Geometry check sheet. Reference: the model listing, model coordinates, mm. Round coordinates to 2 decimals unless told otherwise and drop trailing zeros. Write each loop counter-clockwise with the first axis right and the second up, starting at its lowest first coordinate (ties: lowest second). Pieces come first, ordered by that corner, then holes. Notation, with made-up numbers: M 43,54 L 68,54 A4 cw 68,58 Z; hole C 21,66 d7. An arc over 180 degrees is marked long. Put each result on its own line as item: value. Start each with the question number.
(1) Mould release check, pull along X, two halves, no side actions. Record for faces 1 (the flat face through (18, 1, 3.18)), 2 (the cylindrical face through (-0.54, -2.44, 1.61)): pulls with the +X half, pulls with the -X half, needs draft (parallel to the pull), parting line crosses it, or undercut.
(2) Section check A-A on z = 0.85. Count the separate pieces of the cut face and the enclosed holes in it, then the cut area to 3 significant figures.
(3) Material ranges on probe 1 along Y at (x, z) = (-70, 3.05); probe 2 along Y at (x, z) = (6.1, 1.55); probe 3 along Y at (x, z) = (2, 1), recorded low to high.
(4) Section check B-B on x = 36. Record the cut outline in (y, z).
(5) Gauge pin test, flat ends, axial feed: pin 1 (0.9 mm diameter, centred on x = -69, z = 2, fed in from -Y); pin 2 (1.6 mm diameter, centred on x = -77, z = 2, fed in from +Y); pin 3 (1.5 mm diameter, centred on y = -3.5, z = 1, fed in from +X). Record the tip position at first contact, or that the pin passes through.
from build123d import *

# Parameters (mm, degrees)
SKETCH1_R           = 1.5
BOSS_EXTRUDE1_DEPTH = 3.18
SKETCH2_R           = 2.5
SKETCH2_R_2         = 1.5
CUT_EXTRUDE1_DEPTH  = 20
SKETCH3_R           = 1.5
CUT_EXTRUDE2_DEPTH  = 20
SKETCH5_R           = 1.5
CUT_EXTRUDE4_DEPTH  = 4


with BuildPart() as part:
    # Sketch1 → Boss-Extrude1 (new body)
    with BuildSketch(Plane.XY):
        Polygon((-78.18, 75), (-12.5, 75), (-12.5, 78.18), (12.5, 78.18), (12.5, 75), (78.18, 75), (78.18, 12.5), (75, 12.5), (75, 1.5), (71, 1.5), (71, 4.5), (68, 4.5), (68, 1.5), (65.18, 1.5), (65.18, -1.5), (68, -1.5), (68, -4.5), (71, -4.5), (71, -1.5), (75, -1.5), (75, -12.5), (78.18, -12.5), (78.18, -75), (12.5, -75), (12.5, -78.18), (-12.5, -78.18), (-12.5, -75), (-78.18, -75), (-78.18, -12.5), (-75, -12.5), (-75, -1.5), (-71, -1.5), (-71, -4.5), (-68, -4.5), (-68, -1.5), (-65.18, -1.5), (-65.18, 1.5), (-68, 1.5), (-68, 4.5), (-71, 4.5), (-71, 1.5), (-75, 1.5), (-75, 12.5), (-78.18, 12.5), align=None)
        with Locations(Location((0, -76.59, 0), (0, 0, 180))):
            Circle(SKETCH1_R, mode=Mode.SUBTRACT)
        with Locations(Location((0, 76.59, 0), (0, 0, 180))):
            Circle(SKETCH1_R, mode=Mode.SUBTRACT)
    extrude(amount=BOSS_EXTRUDE1_DEPTH)

    # Sketch2 → Cut-Extrude1 (cut)
    with BuildSketch(Plane.XY.offset(3.18)):
        Circle(SKETCH2_R)
        with Locations((-5, 0)):
            Circle(SKETCH2_R_2)
        with Locations((5, 0)):
            Circle(SKETCH2_R_2)
    extrude(amount=-CUT_EXTRUDE1_DEPTH, mode=Mode.SUBTRACT)

    # Sketch3 → Cut-Extrude2 (cut)
    with BuildSketch(Plane.XY.offset(3.18)):
        with Locations((56.9, -17.847779645)):
            Circle(SKETCH3_R)
        with Locations((58.5, -66.147779645)):
            Circle(SKETCH3_R)
        with Locations((6.1, -33.147779645)):
            Circle(SKETCH3_R)
        with Locations((6.1, -61.047779645)):
            Circle(SKETCH3_R)
    extrude(amount=-CUT_EXTRUDE2_DEPTH, mode=Mode.SUBTRACT)

    # Sketch5 → Cut-Extrude4 (cut)
    with BuildSketch(Plane.XY.offset(3.18)):
        with Locations((14.702943725, 72.697056275)):
            Circle(SKETCH5_R)
        with Locations((72.697056275, 72.697056275)):
            Circle(SKETCH5_R)
        with Locations((14.702943725, -14.697056275)):
            Circle(SKETCH5_R)
        with Locations((72.697056275, -14.697056275)):
            Circle(SKETCH5_R)
    extrude(amount=-CUT_EXTRUDE4_DEPTH, mode=Mode.SUBTRACT)


solid = part.part
Answers follow:
1. face 1: needs draft
1. face 2: undercut
2. separate pieces: 1
2. enclosed holes: 13
2. area: 23,300 mm^2
3. probe 1: y = -75 to -4.5, 4.5 to 75
3. probe 2: y = -78.18 to -62.55, -59.55 to -34.65, -31.65 to -1.02, 1.02 to 78.18
3. probe 3: y = -78.18 to -1.5, 1.5 to 78.18
4. outline: M -75,0 L 75,0 L 75,3.18 L -75,3.18 Z
5. pin 1: stops at y = -75
5. pin 2: stops at y = 75
5. pin 3: stops at x = 75
